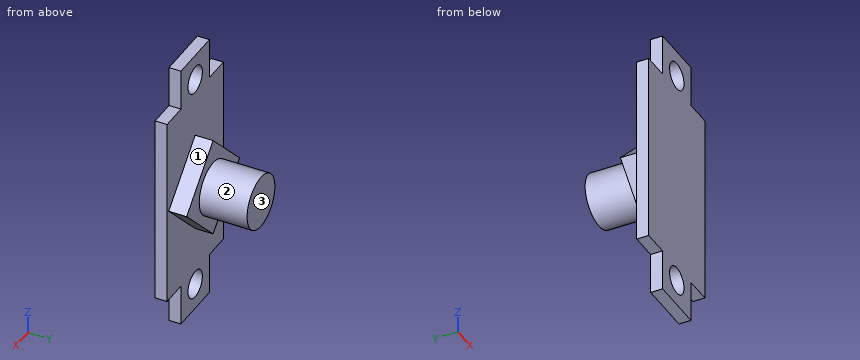
from build123d import *

# Parameters (mm, degrees)
SKETCH1_W           = 2.225
SKETCH1_H           = 16.1
SKETCH1_W_2         = 4.55
SKETCH1_H_2         = 3.45
SKETCH1_R           = 1.15
BOSS_EXTRUDE1_DEPTH = 1
BOSS_EXTRUDE2_DEPTH = 1.5
SKETCH3_R           = 2.226640197
BOSS_EXTRUDE3_DEPTH = 4


with BuildPart() as part:
    # Sketch1 → Boss-Extrude1 (new body)
    # profile 1 of 5: a face of its own
    with BuildSketch(Plane(origin=(0, 0, 0), x_dir=(1, 0, 0), z_dir=(0, 1, 0))):
        with Locations((-3.3875, 0)):
            Rectangle(SKETCH1_W, SKETCH1_H)
    # profile 2 of 5: a face of its own
    with BuildSketch(Plane(origin=(0, 0, 0), x_dir=(1, 0, 0), z_dir=(0, 1, 0))):
        with Locations((0, 9.775)):
            Rectangle(SKETCH1_W_2, SKETCH1_H_2)
        with Locations(Location((0, 9.3, 0), (0, 0, 270))):
            Circle(SKETCH1_R, mode=Mode.SUBTRACT)
    # profile 3 of 5: a face of its own
    with BuildSketch(Plane(origin=(0, 0, 0), x_dir=(1, 0, 0), z_dir=(0, 1, 0))):
        Rectangle(SKETCH1_W_2, SKETCH1_H)
    # profile 4 of 5: a face of its own
    with BuildSketch(Plane(origin=(0, 0, 0), x_dir=(1, 0, 0), z_dir=(0, 1, 0))):
        with Locations((3.3875, 0)):
            Rectangle(SKETCH1_W, SKETCH1_H)
    # profile 5 of 5: a face of its own
    with BuildSketch(Plane(origin=(0, 0, 0), x_dir=(1, 0, 0), z_dir=(0, 1, 0))):
        with Locations((0, -9.775)):
            Rectangle(SKETCH1_W_2, SKETCH1_H_2)
        with Locations(Location((0, -9.3, 0), (0, 0, 270))):
            Circle(SKETCH1_R, mode=Mode.SUBTRACT)
    extrude(amount=BOSS_EXTRUDE1_DEPTH)

    # Sketch2 → Boss-Extrude2 (add)
    with BuildSketch(Plane(origin=(0, 1, 0), x_dir=(1, 0, 0), z_dir=(0, 1, 0))):
        Polygon((0, -4.242640687), (4.242640687, 0), (0, 4.242640687), (-4.242640687, 0), align=None)
    extrude(amount=BOSS_EXTRUDE2_DEPTH)

    # Sketch3 → Boss-Extrude3 (add)
    with BuildSketch(Plane(origin=(0, 2.5, 0), x_dir=(1, 0, 0), z_dir=(0, 1, 0))):
        with Locations(Location((0, 0, 0), (0, 0, 270))):
            Circle(SKETCH3_R)
    extrude(amount=BOSS_EXTRUDE3_DEPTH)


solid = part.part
The model under review builds one solid part; all positions refer to its coordinate system, in mm. Face numbers are marked on the shaded views. A direction names the side the tool comes from. Round coordinates to 2 decimals unless told otherwise and drop trailing zeros. Loops run counter-clockwise (first coordinate to the right, second up) from the corner with the lowest first, then second, coordinate; pieces in that order, holes last. Notation, with made-up numbers: (-4.75, 9) - (26.25, 9) arc R14 ccw to (26.25, 29) - close; hole circle Ø5 at (75.25, 47.5). An arc over 180 degrees is marked (long way). Use CSV: the item, a comma, the result in double quotes.
(1) For line 1 (X direction, y = 0.65, z = 9.3) (3 decimals); line 2 (Y direction, x = 0.5, z = 2.5); line 3 (Y direction, x = -2.5, z = -4), list the stretches that pass through material, from the lowest coordinate up.
Working result:
line 1,"x = -2.275 to -1.15, 1.15 to 2.275"
line 2,"y = 0 to 2.5"
line 3,"y = 0 to 1"
(2) Clearance check with flat-ended pins moving along their axes: P1, Ø0.5, axis at y = 0.5, z = 10, coming from the +X side (3 decimals); P2, Ø3.5, axis at x = 0, z = -9.3, coming from the -Y side; P3, Ø0.8, axis at y = 0.5, z = -10.5, coming from the -X side (3 decimals); P4, Ø1.5, axis at x = -0.5, y = 5.5, coming from the +Z side. State where each tip first meets the part, or that it passes through.
Working result:
P1,"stops at x = 2.275"
P2,"stops at y = 0"
P3,"stops at x = -2.275"
P4,"stops at z = 2.23"
(3) Take a section at A-A, the plane z = 9.3. Give the boundary of the cut face in (x, y) (3 decimals).
Working result:
outline,"(-2.275, 0) - (-1.15, 0) - (-1.15, 1) - (-2.275, 1) - close; (1.15, 0) - (2.275, 0) - (2.275, 1) - (1.15, 1) - close"
(4) Take a section at D-D, the plane x = -2.5. Give the boundary of the cut face in (y, z), plus the area to 3 significant figures.
Working result:
outline,"(0, -8.05) - (1, -8.05) - (1, -1.74) - (2.5, -1.74) - (2.5, 1.74) - (1, 1.74) - (1, 8.05) - (0, 8.05) - close"
area,"21.3 mm^2"
(5) Take a section at C-C, the plane z = -2. Give the boundary of the cut face in (x, y), plus the area to 3 significant figures.
Working result:
outline,"(-4.5, 0) - (4.5, 0) - (4.5, 1) - (2.24, 1) - (2.24, 2.5) - (0.98, 2.5) - (0.98, 6.5) - (-0.98, 6.5) - (-0.98, 2.5) - (-2.24, 2.5) - (-2.24, 1) - (-4.5, 1) - close"
area,"23.6 mm^2"
(6) Machinability: for the marked faces 1, 2 and 3, which of the approach directions +Z, -Z, +X, -X, +Y, -Y give a long, thin tool a straight path to every point of the face, cutting with its end or side? Answer none if there is none.
Working result:
face 1,"+Z, +X, +Y"
face 2,"+Y"
face 3,"+Z, -Z, +X, -X, +Y"
(7) Take a section at B-B, the plane y = 4. Give the boundary of the cut face in (x, z).
Working result:
outline,"circle Ø4.45 at (0, 0)"
